from build123d import *

# Parameters (mm, degrees)
SKETCH1_R           = 13
BOSS_EXTRUDE2_DEPTH = 2
SKETCH2_R           = 13
SKETCH2_R_2         = 12
BOSS_EXTRUDE3_DEPTH = 15
SKETCH3_R           = 5
CUT_EXTRUDE1_DEPTH  = 15


with BuildPart() as part:
    # Sketch1 → Boss-Extrude2 (new body)
    with BuildSketch(Plane(origin=(0, 0, 0), x_dir=(1, 0, 0), z_dir=(0, 1, 0))):
        with Locations(Location((0, 0, 0), (0, 0, 270))):
            Circle(SKETCH1_R)
    extrude(amount=BOSS_EXTRUDE2_DEPTH)

    # Sketch2 → Boss-Extrude3 (add)
    with BuildSketch(Plane(origin=(0, 2, 0), x_dir=(1, 0, 0), z_dir=(0, 1, 0))):
        with Locations(Location((0, 0, 0), (0, 0, 270))):
            Circle(SKETCH2_R)
        with Locations(Location((0, 0, 0), (0, 0, 270))):
            Circle(SKETCH2_R_2, mode=Mode.SUBTRACT)
    extrude(amount=BOSS_EXTRUDE3_DEPTH)

    # Sketch3 → Cut-Extrude1 (cut)
    with BuildSketch(Plane.XZ):
        with Locations(Location((0, 0, 0), (0, 0, 270))):
            Circle(SKETCH3_R)
    extrude(amount=-CUT_EXTRUDE1_DEPTH, mode=Mode.SUBTRACT)


solid = part.part
The listing builds one solid part. Answer for the finished solid, in the listing's coordinates (mm). Coordinates: 2 decimals unless noted, no trailing zeros. Write each loop counter-clockwise with the first axis right and the second up, starting at its lowest first coordinate (ties: lowest second). Pieces come first, ordered by that corner, then holes. Notation, with made-up numbers: (21, 31) - (43, 31) arc R3 cw to (43, 35) - close; hole circle Ø7 at (72.25, 3.25). An arc over 180 degrees is marked (long way). Answer as CSV lines item,"result".
1. Straight lines are drawn through the part: line 1 (X direction, y = 6.5, z = 0.25); line 2 (X direction, y = 1.45, z = 0); line 3 (Z direction, x = -5.5, y = 3.25). For each, find the intervals that lie inside material, in ascending order. Write a range as [from, to].
Computed values:
line 1,"x = [-13, -12], [12, 13]"
line 2,"x = [-13, -5], [5, 13]"
line 3,"z = [-11.78, -10.67], [10.67, 11.78]"
2. Given P1, Ø1, axis at y = 8, z = 2, coming from the +X side; P2, Ø6, axis at x = -5, z = 6.5, coming from the +Y side; P3, Ø4, axis at x = 7.5, y = 12.5, coming from the -Z side, each flat-ended and moving along its own axis, determine where each tip first touches the part or whether it passes through.
Computed values:
P1,"stops at x = 12.91"
P2,"stops at y = 2"
P3,"stops at z = -11.78"
3. Find section C-C (y = 7.25). Give the vertices of the cut face in (x, z).
Computed values:
outline,"circle Ø26 at (0, 0); hole circle Ø24 at (0, 0)"
4. Find section A-A (z = 0). Give the vertices of the cut face in (x, y).
Computed values:
outline,"(-13, 0) - (-5, 0) - (-5, 2) - (-12, 2) - (-12, 17) - (-13, 17) - close; (5, 0) - (13, 0) - (13, 17) - (12, 17) - (12, 2) - (5, 2) - close"
5. Find section B-B (x = 0). Give the vertices of the cut face in (y, z), plus the area to 3 significant figures.
Computed values:
outline,"(0, -13) - (17, -13) - (17, -12) - (2, -12) - (2, -5) - (0, -5) - close; (0, 5) - (2, 5) - (2, 12) - (17, 12) - (17, 13) - (0, 13) - close"
area,"62.0 mm²"
6. Find section D-D (x = -7.5). Give the vertices of the cut face in (y, z).
Computed values:
outline,"(0, -10.62) - (17, -10.62) - (17, -9.37) - (2, -9.37) - (2, 9.37) - (17, 9.37) - (17, 10.62) - (0, 10.62) - close"
7. Determine the mould class of faces 1 (the cylindrical face through (3.604, 9.395, 11.446)), 2 (the flat face through (0, 0, 6)), 3 (the cylindrical face through (-7.91, 8.381, -10.316)), 4 (the flat face through (0.2, 2, 5.2)) for opening direction X: +X half, -X half, draft (parallel to the pull), parting line (faces both ways), or undercut.
Computed values:
face 1,"undercut"
face 2,"draft"
face 3,"parting line"
face 4,"undercut"
